from build123d import *

# Parameters (mm, degrees)
SKETCH_1_W      = 6.2
SKETCH_1_H      = 1.3
SKETCH_1_W_2    = 1.3
SKETCH_1_H_2    = 6.2
SKETCH_1_W_3    = 10.5
SKETCH_1_H_3    = 10.5
SKETCH_1_R      = 3.4
EXTRUDE_2_DEPTH = 500


with BuildPart() as part:
    # 草图1 → 凸台-拉伸2 (new body)
    with BuildSketch(Plane(origin=(0, 0, 0), x_dir=(1, 0, 0), z_dir=(0, 1, 0))):
        with Locations((-7.3, -19.35)):
            Rectangle(SKETCH_1_W, SKETCH_1_H)
        with BuildLine():
            Line((-18.7, -10.4), (-20, -10.4))
            Line((-20, -10.4), (-20, -16.079155302))
            ThreePointArc((-20, -16.079155302), (-18.851611176, -18.851611176), (-16.079155302, -20))
            Line((-16.079155302, -20), (-10.4, -20))
            Line((-10.4, -20), (-10.4, -18.7))
            Line((-10.4, -18.7), (-10.4, -11.319238816))
            Line((-10.4, -11.319238816), (-10.4, -10.4))
            Line((-10.4, -10.4), (-11.319238816, -10.4))
            Line((-11.319238816, -10.4), (-18.7, -10.4))
        make_face()
        Polygon((-18.7, -15.2), (-18.7, -11.7), (-15.2, -11.7), (-11.7, -11.7), (-11.7, -15.2), (-11.7, -18.7), (-15.2, -18.7), (-18.7, -18.7), align=None, mode=Mode.SUBTRACT)
        with Locations((-19.35, -7.3)):
            Rectangle(SKETCH_1_W_2, SKETCH_1_H_2)
        with BuildLine():
            ThreePointArc((-15.2, -18.7), (-17.674873734, -17.674873734), (-18.7, -15.2))
            Line((-18.7, -15.2), (-18.7, -18.7))
            Line((-18.7, -18.7), (-15.2, -18.7))
        make_face()
        Polygon((-5.25, -5.25), (-5.25, -4.330761184), (-11.319238816, -10.4), (-10.4, -10.4), (-10.4, -11.319238816), (-4.330761184, -5.25), align=None)
        Rectangle(SKETCH_1_W_3, SKETCH_1_H_3)
        with Locations(Location((0, 0, 0), (0, 0, 270))):
            Circle(SKETCH_1_R, mode=Mode.SUBTRACT)
        Polygon((11.319238816, -10.4), (5.25, -4.330761184), (5.25, -5.25), (4.330761184, -5.25), (10.4, -11.319238816), (10.4, -10.4), align=None)
        Polygon((10.4, 11.319238816), (4.330761184, 5.25), (5.25, 5.25), (5.25, 4.330761184), (11.319238816, 10.4), (10.4, 10.4), align=None)
        Polygon((-4.330761184, 5.25), (-10.4, 11.319238816), (-10.4, 10.4), (-11.319238816, 10.4), (-5.25, 4.330761184), (-5.25, 5.25), align=None)
        with BuildLine():
            Line((18.7, -10.4), (11.319238816, -10.4))
            Line((11.319238816, -10.4), (10.4, -10.4))
            Line((10.4, -10.4), (10.4, -11.319238816))
            Line((10.4, -11.319238816), (10.4, -18.7))
            Line((10.4, -18.7), (10.4, -20))
            Line((10.4, -20), (16.079155302, -20))
            ThreePointArc((16.079155302, -20), (18.851611176, -18.851611176), (20, -16.079155302))
            Line((20, -16.079155302), (20, -10.4))
            Line((20, -10.4), (18.7, -10.4))
        make_face()
        Polygon((15.2, -11.7), (18.7, -11.7), (18.7, -15.2), (18.7, -18.7), (15.2, -18.7), (11.7, -18.7), (11.7, -15.2), (11.7, -11.7), align=None, mode=Mode.SUBTRACT)
        with BuildLine():
            Line((18.7, -18.7), (18.7, -15.2))
            ThreePointArc((18.7, -15.2), (17.674873734, -17.674873734), (15.2, -18.7))
            Line((15.2, -18.7), (18.7, -18.7))
        make_face()
        with BuildLine():
            Line((16.079155302, 20), (10.4, 20))
            Line((10.4, 20), (10.4, 18.7))
            Line((10.4, 18.7), (10.4, 11.319238816))
            Line((10.4, 11.319238816), (10.4, 10.4))
            Line((10.4, 10.4), (11.319238816, 10.4))
            Line((11.319238816, 10.4), (18.7, 10.4))
            Line((18.7, 10.4), (20, 10.4))
            Line((20, 10.4), (20, 16.079155302))
            ThreePointArc((20, 16.079155302), (18.851611176, 18.851611176), (16.079155302, 20))
        make_face()
        Polygon((15.2, 18.7), (18.7, 18.7), (18.7, 15.2), (18.7, 11.7), (15.2, 11.7), (11.7, 11.7), (11.7, 15.2), (11.7, 18.7), align=None, mode=Mode.SUBTRACT)
        with BuildLine():
            Line((18.7, 15.2), (18.7, 18.7))
            Line((18.7, 18.7), (15.2, 18.7))
            ThreePointArc((15.2, 18.7), (17.674873734, 17.674873734), (18.7, 15.2))
        make_face()
        with BuildLine():
            Line((-10.4, 20), (-16.079155302, 20))
            ThreePointArc((-16.079155302, 20), (-18.851611176, 18.851611176), (-20, 16.079155302))
            Line((-20, 16.079155302), (-20, 10.4))
            Line((-20, 10.4), (-18.7, 10.4))
            Line((-18.7, 10.4), (-11.319238816, 10.4))
            Line((-11.319238816, 10.4), (-10.4, 10.4))
            Line((-10.4, 10.4), (-10.4, 11.319238816))
            Line((-10.4, 11.319238816), (-10.4, 18.7))
            Line((-10.4, 18.7), (-10.4, 20))
        make_face()
        Polygon((-15.2, 11.7), (-18.7, 11.7), (-18.7, 15.2), (-18.7, 18.7), (-15.2, 18.7), (-11.7, 18.7), (-11.7, 15.2), (-11.7, 11.7), align=None, mode=Mode.SUBTRACT)
        with BuildLine():
            Line((-18.7, 18.7), (-18.7, 15.2))
            ThreePointArc((-18.7, 15.2), (-17.674873734, 17.674873734), (-15.2, 18.7))
            Line((-15.2, 18.7), (-18.7, 18.7))
        make_face()
        with Locations((-7.3, 19.35)):
            Rectangle(SKETCH_1_W, SKETCH_1_H)
        with Locations((7.3, 19.35)):
            Rectangle(SKETCH_1_W, SKETCH_1_H)
        with Locations((19.35, 7.3)):
            Rectangle(SKETCH_1_W_2, SKETCH_1_H_2)
        with Locations((-19.35, 7.3)):
            Rectangle(SKETCH_1_W_2, SKETCH_1_H_2)
        with Locations((19.35, -7.3)):
            Rectangle(SKETCH_1_W_2, SKETCH_1_H_2)
        with Locations((7.3, -19.35)):
            Rectangle(SKETCH_1_W, SKETCH_1_H)
    extrude(amount=EXTRUDE_2_DEPTH)


solid = part.part
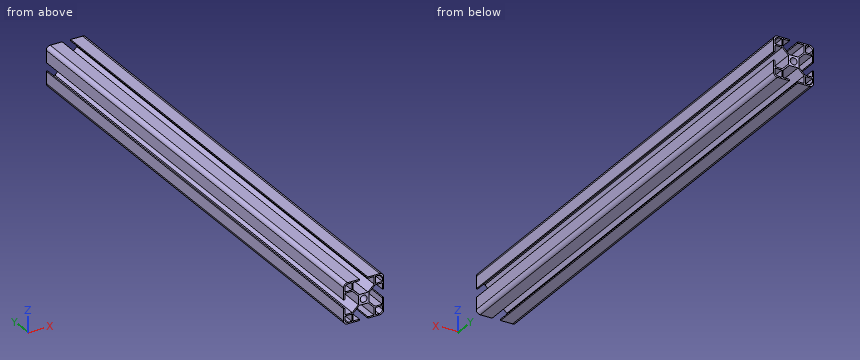
The model under review builds one solid part; all positions refer to its coordinate system, in mm. Give positions to 0.01 mm unless a question says otherwise; leave off trailing zeros.
1. Wall thickness on L1, parallel to X at y = 474.5, z = 15.5; L2, parallel to Z at x = -16, y = 81; L3, parallel to Z at x = -12, y = 301: over which ranges is each line inside the solid? List them lowest first.
2. For P1, Ø8, axis at x = 8, z = -13.5, coming from the +Y side, flat-tipped, find the tip position at first contact; note if it passes through.
3. Add section A-A, the plane y = 111. Count the separate pieces of the cut face and the enclosed holes in it, plus the area to 3 significant figures.
Worked answers:
1. L1: x = -20 to -18.69, -11.7 to -10.4, 10.4 to 11.7, 18.69 to 20
1. L2: z = -20 to -18.61, -11.7 to -10.4, 10.4 to 11.7, 18.61 to 20
1. L3: z = -20 to -18.7, -11.7 to -10.4, 10.4 to 11.7, 18.7 to 20
2. P1: stops at y = 500
3. separate pieces: 1
3. enclosed holes: 5
3. area: 350 mm2
